Design review of the part built by this model. Coordinates are the model's own, in mm. Round coordinates to 2 decimals unless told otherwise and drop trailing zeros. Loops run counter-clockwise (first coordinate to the right, second up) from the corner with the lowest first, then second, coordinate; pieces in that order, holes last. Notation, with made-up numbers: (19, -37) - (23, -37) arc R23 cw to (23, -18) - close; hole circle Ø3 at (9.5, -20). An arc over 180 degrees is marked (long way). Use one line per item in the form item = value. Start each with the question number.
(1) We need section A-A, the plane z = 569. Write out the cut boundary in (x, y).
(2) Wall thickness on probe 1 along Z at (x, y) = (-5, 3.5); probe 2 along Z at (x, y) = (-25, 3); probe 3 along X at (y, z) = (2, 51): over which ranges is each line inside the solid? List them lowest first. Write a range as [from, to].
(3) For pin 1 (1 mm diameter, centred on x = 15.5, y = 11, fed in from -Z); pin 2 (6 mm diameter, centred on y = 10, z = 485, fed in from -X); pin 3 (10 mm diameter, centred on x = -16.5, y = -5, fed in from -Z); pin 4 (10 mm diameter, centred on y = -16, z = 423, fed in from -X), all flat-tipped, find the tip position at first contact; note any pin that passes through.
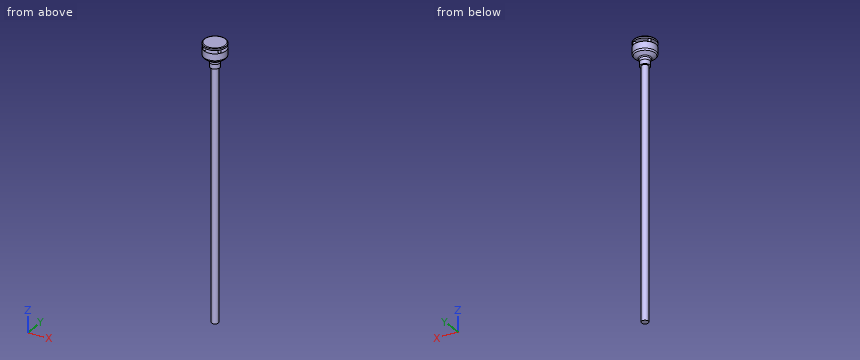
Autodesk Inventor part; units mm, degrees
ref_plane "YZ Plane" through (0, 0, 0) normal (1, 0, 0) x (0, 1, 0)
ref_plane "XZ Plane" through (0, 0, 0) normal (0, 1, 0) x (-1, 0, 0)
ref_plane "XY Plane" through (0, 0, 0) normal (0, 0, 1) x (1, 0, 0)
sketch "Sketch1" plane through (0, 0, 0) normal (0, 0, 1) x (1, 0, 0)
  circle A0 centre (0, 0) radius 9
  dimension "d0" = 18
extrude "Extrusion1" add sketch "Sketch1" along normal blind 700
sketch "Sketch2" plane through (0, 0, 700) normal (0, 0, 1) x (1, 0, 0)
  circle A0 centre (0, 0) radius 9
  circle A1 centre (0, 0) radius 30
  circle A2 centre (0, 0) radius 13
  dimension "d3" = 60
  dimension "d33" = 26
extrude "Extrusion2" add sketch "Sketch2" along normal blind 30 contours A0 | A1 | A2
sketch "Sketch3" plane through (0, 0, 730) normal (0, 0, 1) x (1, 0, 0)
  circle A0 centre (0, 0) radius 30
  line L0 (-24.495, 17.3203) -> (0, 0) construction
  line L1 (24.495, -17.3203) -> (0, 0) construction
  line L2 (0, 0) -> (17.3203, 24.495) construction
  line L3 (0, 0) -> (-17.3203, -24.495) construction
  circle A1 centre (-21.6666, 15.3203) radius 3
  circle A2 centre (-15.3203, -21.6666) radius 3
  circle A3 centre (21.6666, -15.3203) radius 3
  circle A4 centre (15.3203, 21.6666) radius 3
  dimension "d18" = 6
  dimension "d19" = 2
  dimension "d22" = 360
extrude "Extrusion3" add sketch "Sketch3" along normal blind 8.6 contours A1 | A2 | A3 | A4
sketch "Sketch4" plane through (0, 0, 738.6) normal (0, 0, 1) x (1, 0, 0)
  circle A0 centre (0, 0) radius 30
  dimension "d9" = 60
extrude "Extrusion4" add sketch "Sketch4" along normal blind 6
chamfer "Chamfer2" distance 15.25 angle 30 1 edges at (-30, 0, 700) measured on face at (22.6222, -3.1111, 700)
fillet "Fillet5" radius 5 1 edges at (-30, 0, 708.8046)
extrude "Extrusion5" add sketch "Sketch2" against normal blind 20 contours A2
fillet "Fillet7" radius 20 1 edges at (-13, 0, 700)
fillet "Fillet8" radius 5 1 edges at (-14.75, 0, 700)
fillet "Fillet9" radius 2 1 edges at (-30, 0, 744.6)
properties part number "anemo"
Data:
q1.outline = circle Ø18 at (0, 0)
q2.probe_1 = [0, 730], [738.6, 744.6]
q2.probe_2 = [706.02, 730], [738.6, 744.6]
q2.probe_3 = [-8.77, 8.77]
q3.pin_1 = 702.17
q3.pin_2 = -5.66
q3.pin_3 = 680
q3.pin_4 = through
